Model file for the job. Use its own axes, mm. A direction names the side the tool comes from. Coordinates: 2 decimals unless noted, no trailing zeros. Order: outer loops, then holes, each group sorted by start corner. A loop starts at its lowest first (then second) coordinate and runs counter-clockwise, first axis right, second up. Notation, with made-up numbers: (18, 34.25) -> (41, 34.25) arc R26 cw to (41, 64.25) -> close; hole circle Ø2 at (-5.75, -29.75). An arc over 180 degrees is marked (long way). Return JSON: item names as keys, results as strings. Group by question number.
1) Cut at A-A (x = 20). Write the cut outline in (y, z).
2) Flat gauge pin, fed straight in: pin 1 (6.5 mm diameter, centred on x = 19, z = 9, fed in from +Y). Where does the tip first touch, or does it go through?
3) Cut at D-D (z = 1). Write the cut outline in (x, y).
4) Probe line 1 (Z direction, x = 32, y = 75.5); line 2 (X direction, y = 28, z = 2.5); line 3 (X direction, y = 68.5, z = 13.5). List the from-to ranges inside material, lowest first.
5) Pull direction Z, two halves, no side cores. Call faces 4 (the cylindrical face through (20.79, 78.69, 16.48)), 5 (the flat face through (28, 71, 9)), 6 (the flat face through (20, 47, 0)), 7 (the cylindrical face through (4.27, 1.04, 8.38)): +Z half, -Z half, draft (parallel to the pull), parting line (faces both ways), or undercut.
6) Cut at C-C (y = 17.5). Write the cut outline in (x, z), and give its area (3 significant figures).
7) Which spindle directions (+Z, -Z, +X, -X, +Y, -Y) get a long thin tool onto all of the face, cutting with end or side? Do faces 1 (the flat face through (3.77, 17.86, 11.27)), 2 (the flat face through (5, 17, 5)), 3 (the flat face through (21, 77, 2)). Say none if no direction does.
8) Cut at B-B (z = 8.5). Write the cut outline in (x, y), and give its area (3 significant figures).
from build123d import *

# Parameters (mm, degrees)
SKETCH1_W             = 5
SKETCH1_H             = 17
BOSS_EXTRUDE1_DEPTH   = 80
BOSS_EXTRUDE1_2_DEPTH = 80
CUT_EXTRUDE1_DEPTH    = 2.5
BOSS_EXTRUDE2_REACH   = 91.359
SKETCH5_W             = 3
SKETCH5_H             = 13
CUT_EXTRUDE2_DEPTH    = 5
FILLET1_R             = 3
FILLET2_R             = 3
SKETCH6_R             = 1.5
CUT_EXTRUDE3_DEPTH    = 90.358827208
BOSS_EXTRUDE3_REACH   = 91.359
SKETCH7_W             = 17
SKETCH7_H             = 37.482200285


with BuildPart() as part:
    # Sketch1 → Boss-Extrude1 (new body)
    with BuildSketch(Plane(origin=(0, 0, 0), x_dir=(1, 0, 0), z_dir=(0, 1, 0))):
        with Locations((2.5, -8.5)):
            Rectangle(SKETCH1_W, SKETCH1_H)
    extrude(amount=BOSS_EXTRUDE1_DEPTH)

    # Sketch2 → Cut-Extrude1 (cut)
    with BuildSketch(Plane(origin=(5, 0, 0), x_dir=(0, 0, -1), z_dir=(1, 0, 0))):
        with BuildLine():
            Line((-10.75, 25.267799715), (-11.807189139, 10.25))
            ThreePointArc((-11.807189139, 10.25), (-8.5, 12), (-5.192810861, 10.25))
            Line((-5.192810861, 10.25), (-6.25, 25.267799715))
            ThreePointArc((-6.25, 25.267799715), (-8.5, 27.517799715), (-10.75, 25.267799715))
        make_face()
        with BuildLine():
            ThreePointArc((-5.192810861, 10.25), (-8.5, 12), (-11.807189139, 10.25))
            Line((-11.807189139, 10.25), (-11.807189139, 5.75))
            ThreePointArc((-11.807189139, 5.75), (-8.5, 4), (-5.192810861, 5.75))
            Line((-5.192810861, 5.75), (-5.192810861, 10.25))
        make_face()
        with BuildLine():
            Line((-11.807189139, 5.75), (-11.807189139, 10.25))
            ThreePointArc((-11.807189139, 10.25), (-12.5, 8), (-11.807189139, 5.75))
        make_face()
        with BuildLine():
            ThreePointArc((-4.5, 8), (-4.677124344, 9.177124344), (-5.192810861, 10.25))
            Line((-5.192810861, 10.25), (-5.192810861, 5.75))
            ThreePointArc((-5.192810861, 5.75), (-4.677124344, 6.822875656), (-4.5, 8))
        make_face()
    extrude(amount=-CUT_EXTRUDE1_DEPTH, mode=Mode.SUBTRACT)


with BuildPart() as body_2:
    # Sketch1 → Boss-Extrude1 2 (new body)
    with BuildSketch(Plane(origin=(0, 0, 0), x_dir=(1, 0, 0), z_dir=(0, 1, 0))):
        with Locations((38.5, -8.5)):
            Rectangle(SKETCH1_W, SKETCH1_H)
    extrude(amount=BOSS_EXTRUDE1_2_DEPTH)


    # Sketch4 → Boss-Extrude2 (add, up to next)
    with BuildSketch(Plane.ZY.offset(-36), mode=Mode.PRIVATE) as boss_extrude2_sk1:
        Polygon((2, 73), (15, 73), (15, 80), (17, 80), (17, 72), (17, 68), (0, 68), (0, 72), (0, 80), (2, 80), align=None)
    boss_extrude2_tool1 = extrude(boss_extrude2_sk1.sketch, amount=BOSS_EXTRUDE2_REACH, mode=Mode.PRIVATE) - part.part
    add(boss_extrude2_tool1.solids().sort_by_distance((36, 71.986726, 8.5))[0])

    # Sketch5 → Cut-Extrude2 (cut)
    with BuildSketch(Plane(origin=(0, 73, 0), x_dir=(1, 0, 0), z_dir=(0, 1, 0))):
        with Locations((29.5, -8.5)):
            Rectangle(SKETCH5_W, SKETCH5_H)
    extrude(amount=-CUT_EXTRUDE2_DEPTH, mode=Mode.SUBTRACT)

    # Fillet1
    # the kernel refuses this fillet: 3 mm, written as the material it takes off along each edge
    with BuildSketch(Plane(origin=(36, 0, 24.5), x_dir=(0, 1, 0), z_dir=(0, 0, -1)), Plane(origin=(41, 0, -7.5), x_dir=(0, 1, 0), z_dir=(0, 0, 1)), Plane(origin=(41, 80, -7.5), x_dir=(-1, 0, 0), z_dir=(0, 0, 1))) as fillet1_piece_1:
        with BuildLine():
            CenterArc((FILLET1_R, FILLET1_R), FILLET1_R, 180, 90)
            Line((0, FILLET1_R), (0, 0))
            Line((0, 0), (FILLET1_R, 0))
        make_face()
    extrude(amount=32, mode=Mode.SUBTRACT)
    with BuildSketch(Plane(origin=(-2.5, 80, 17), x_dir=(0, 0, -1), z_dir=(1, 0, 0)), Plane(origin=(48.5, 80, 0), x_dir=(0, 0, 1), z_dir=(-1, 0, 0))) as fillet1_piece_2:
        with BuildLine():
            CenterArc((FILLET1_R, -FILLET1_R), FILLET1_R, 90, 90)
            Line((0, -FILLET1_R), (0, 0))
            Line((0, 0), (FILLET1_R, 0))
        make_face()
    extrude(amount=51, mode=Mode.SUBTRACT)

    # Sketch6 → Cut-Extrude3 (cut, through all)
    with BuildSketch(Plane.ZY.offset(-36)):
        with Locations((8.686376561, 8.041960108)):
            Circle(SKETCH6_R)
    extrude(amount=-CUT_EXTRUDE3_DEPTH, mode=Mode.SUBTRACT)

    # Sketch7 → Boss-Extrude3 (add, up to next)
    with BuildSketch(Plane(origin=(5, 0, 0), x_dir=(0, 0, -1), z_dir=(1, 0, 0)), mode=Mode.PRIVATE) as boss_extrude3_sk1:
        with Locations((-8.5, 49.258899857)):
            Rectangle(SKETCH7_W, SKETCH7_H)
    boss_extrude3_tool1 = extrude(boss_extrude3_sk1.sketch, amount=BOSS_EXTRUDE3_REACH, mode=Mode.PRIVATE) - body_2.part


with BuildPart() as part_1:
    add(part.part)

    # Fillet2
    # the kernel refuses this fillet: 3 mm, written as the material it takes off along each edge
    with BuildSketch(Plane(origin=(0, 0, 24.5), x_dir=(0, 1, 0), z_dir=(0, 0, -1)), Plane(origin=(5, 0, -7.5), x_dir=(0, 1, 0), z_dir=(0, 0, 1))) as fillet2_piece_1:
        with BuildLine():
            CenterArc((FILLET2_R, FILLET2_R), FILLET2_R, 180, 90)
            Line((0, FILLET2_R), (0, 0))
            Line((0, 0), (FILLET2_R, 0))
        make_face()
    extrude(amount=32, mode=Mode.SUBTRACT)
    with BuildSketch(Plane(origin=(12.5, 80, 17), x_dir=(0, 0, -1), z_dir=(-1, 0, 0))) as fillet2_piece_2:
        with BuildLine():
            CenterArc((FILLET2_R, FILLET2_R), FILLET2_R, 180, 90)
            Line((0, FILLET2_R), (0, 0))
            Line((0, 0), (FILLET2_R, 0))
        make_face()
    extrude(amount=20, mode=Mode.SUBTRACT)
    with BuildSketch(Plane(origin=(0, 80, 24.5), x_dir=(0, -1, 0), z_dir=(0, 0, -1))) as fillet2_piece_3:
        with BuildLine():
            CenterArc((FILLET2_R, -FILLET2_R), FILLET2_R, 90, 90)
            Line((0, -FILLET2_R), (0, 0))
            Line((0, 0), (FILLET2_R, 0))
        make_face()
    extrude(amount=32, mode=Mode.SUBTRACT)
    with BuildSketch(Plane(origin=(-7.5, 80, 0), x_dir=(0, -1, 0), z_dir=(1, 0, 0))) as fillet2_piece_4:
        with BuildLine():
            CenterArc((FILLET2_R, -FILLET2_R), FILLET2_R, 90, 90)
            Line((0, -FILLET2_R), (0, 0))
            Line((0, 0), (FILLET2_R, 0))
        make_face()
    extrude(amount=20, mode=Mode.SUBTRACT)


with BuildPart() as body_2_1:
    add(body_2.part)

    add(part_1.part)  # Boss-Extrude3 merges part
    add(boss_extrude3_tool1.solids().sort_by_distance((5, 49.2589, 8.5))[0])


solid = body_2_1.part
Answers below:
{
 "1": {"outline": "(30.52, 0) -> (77, 0) arc R3 ccw to (79.83, 2) -> (73, 2) -> (73, 15) -> (79.83, 15) arc R3 ccw to (77, 17) -> (30.52, 17) -> close"},
 "2": {"pin 1": "stops at y = 73"},
 "3": {"outline": "(0, 3) arc R3 ccw to (2.5, 0.04) arc R3 ccw to (5, 3) -> (5, 30.52) -> (36, 30.52) -> (36, 3) arc R3 ccw to (38.5, 0.04) arc R3 ccw to (41, 3) -> (41, 77) arc R3 ccw to (40, 79.24) -> (1, 79.24) arc R3 ccw to (0, 77) -> close"},
 "4": {"line 1": "z = 0 to 2, 15 to 17", "line 2": "x = 0 to 5, 36 to 41", "line 3": "x = 0 to 28, 31 to 41"},
 "5": {"face 4": "+Z half", "face 5": "undercut", "face 6": "-Z half", "face 7": "draft"},
 "6": {"outline": "(0, 0) -> (5, 0) -> (5, 5.7) -> (2.5, 5.7) -> (2.5, 11.3) -> (5, 11.3) -> (5, 17) -> (0, 17) -> close; (36, 0) -> (41, 0) -> (41, 17) -> (36, 17) -> close", "area": "156 mm^2"},
 "7": {"face 1": "none", "face 2": "+Z, -Z, -Y", "face 3": "+Y"},
 "8": {"outline": "(0, 3) arc R3 ccw to (2.5, 0.04) arc R3 ccw to (5, 3) -> (5, 4) -> (2.5, 4) -> (2.5, 27.52) -> (5, 27.52) -> (5, 30.52) -> (36, 30.52) -> (36, 9.53) -> (41, 9.53) -> (41, 77) arc R3 ccw to (38, 80) -> (36, 80) -> (36, 73) -> (31, 73) -> (31, 68) -> (28, 68) -> (28, 73) -> (5, 73) -> (5, 80) -> (3, 80) arc R3 ccw to (0, 77) -> close; (36, 3) arc R3 ccw to (38.5, 0.04) arc R3 ccw to (41, 3) -> (41, 6.55) -> (36, 6.55) -> close", "area": "2,020 mm^2"}
}
